Could you check a few things on this model? Use its own coordinates, in mm. A direction names the side the tool comes from. Give positions to 0.01 mm unless a question says otherwise; leave off trailing zeros. Write each loop counter-clockwise with the first axis right and the second up, starting at its lowest first coordinate (ties: lowest second). Pieces come first, ordered by that corner, then holes. Notation, with made-up numbers: (6, -14) - (56, -14) arc R23 cw to (56, 10) - close; hole circle Ø1 at (19, 56.5). An arc over 180 degrees is marked (long way). Answer in a Markdown table with one row per item.
from build123d import *

# Parameters (mm, degrees)
BOSS_EXTRUDE2_DEPTH = 5
SKETCH5_R           = 1
CUT_EXTRUDE2_DEPTH  = 5
SKETCH6_W           = 30.946174702
SKETCH6_H           = 5
BOSS_EXTRUDE3_DEPTH = 30
SKETCH10_R          = 10
CUT_EXTRUDE3_DEPTH  = 30


with BuildPart() as part:
    # Sketch3 → Boss-Extrude2 (new body)
    with BuildSketch(Plane(origin=(0, 0, 0), x_dir=(0, 0, -1), z_dir=(1, 0, 0))):
        with BuildLine():
            Line((15.473087351, -60.931791337), (-15.473087351, -60.931791337))
            Line((-15.473087351, -60.931791337), (-15.473087351, -100.931791337))
            ThreePointArc((-15.473087351, -100.931791337), (0, -116.404878688), (15.473087351, -100.931791337))
            Line((15.473087351, -100.931791337), (15.473087351, -60.931791337))
        make_face()
    extrude(amount=BOSS_EXTRUDE2_DEPTH)

    # Sketch5 → Cut-Extrude2 (cut)
    with BuildSketch(Plane.ZY):
        with Locations((0, -100.931791337)):
            Circle(SKETCH5_R)
    extrude(amount=-CUT_EXTRUDE2_DEPTH, mode=Mode.SUBTRACT)

    # Sketch6 → Boss-Extrude3 (add)
    with BuildSketch(Plane.ZY):
        with Locations((0, -63.431791337)):
            Rectangle(SKETCH6_W, SKETCH6_H)
    extrude(amount=BOSS_EXTRUDE3_DEPTH)

    # Sketch10 → Cut-Extrude3 (cut)
    with BuildSketch(Plane.XZ.offset(65.931791337)):
        with Locations(Location((-15, 0, 0), (0, 0, 270))):
            Circle(SKETCH10_R)
    extrude(amount=-CUT_EXTRUDE3_DEPTH, mode=Mode.SUBTRACT)


solid = part.part
1) If I drill on line 1 (X direction, y = -64.3, z = 0); line 2 (Y direction, x = 3.6, z = 0); line 3 (X direction, y = -90, z = 4), over which ranges is the centre line in solid material (lowest first)?
Check values:
| item | result |
|---|---|
| line 1 | x = -30 to -25, -5 to 5 |
| line 2 | y = -116.4 to -101.93, -99.93 to -60.93 |
| line 3 | x = 0 to 5 |
2) We'd pull the mould along X, two halves only. Please class faces 1 (the face through (2.5, -101.8, 0.5)), 2 (the face through (5, -88, 0)), 3 (the face through (-5.085, -63.467, 1.302)): +X half, -X half, draft (parallel to the pull), parting line (faces both ways), or undercut.
Check values:
| item | result |
|---|---|
| face 1 | draft |
| face 2 | +X half |
| face 3 | undercut |
3) Will these pins go through, and if not, where does the flat tip stop? P1, Ø1.8, axis at y = -100.93, z = 0, coming from the -X side; P2, Ø1, axis at y = -100.5, z = -3.5, coming from the -X side; P3, Ø5, axis at x = -11.5, z = 9.5, coming from the -Y side.
Check values:
| item | result |
|---|---|
| P1 | passes through |
| P2 | stops at x = 0 |
| P3 | stops at y = -65.93 |
4) Imagine slicing it at A-A (x = -15). List the corners of the cut face in (y, z) for me, then the cut area to 3 significant figures.
Check values:
| item | result |
|---|---|
| outline | (-65.93, -15.47) - (-60.93, -15.47) - (-60.93, -10) - (-65.93, -10) - close; (-65.93, 10) - (-60.93, 10) - (-60.93, 15.47) - (-65.93, 15.47) - close |
| area | 54.7 mm2 |
5) Imagine slicing it at C-C (z = 6). List the corners of the cut face in (x, y) for me.
Check values:
| item | result |
|---|---|
| outline | (-30, -65.93) - (-23, -65.93) - (-23, -60.93) - (-30, -60.93) - close; (-7, -65.93) - (0, -65.93) - (0, -115.19) - (5, -115.19) - (5, -60.93) - (-7, -60.93) - close |
6) On a 3-axis mill with a long thin cutter (end or side, diameter ignored), from which of +Z, -Z, +X, -X, +Y, -Y can I reach the whole of each face in a straight line? I mean faces 4 (the face through (0, -91, 0)), 5 (the face through (2.5, -116.4, 0.3)). Say none if no direction works.
Check values:
| item | result |
|---|---|
| face 4 | +Z, -Z, -X, -Y |
| face 5 | +X, -X, -Y |
7) Imagine slicing it at B-B (z = 0). List the corners of the cut face in (x, y) for me.
Check values:
| item | result |
|---|---|
| outline | (-30, -65.93) - (-25, -65.93) - (-25, -60.93) - (-30, -60.93) - close; (-5, -65.93) - (0, -65.93) - (0, -99.93) - (5, -99.93) - (5, -60.93) - (-5, -60.93) - close; (0, -116.4) - (5, -116.4) - (5, -101.93) - (0, -101.93) - close |
8) Imagine slicing it at D-D (y = -79). List the corners of the cut face in (x, z) for me, then the cut area to 3 significant figures.
Check values:
| item | result |
|---|---|
| outline | (0, -15.47) - (5, -15.47) - (5, 15.47) - (0, 15.47) - close |
| area | 155 mm2 |
